Read the model definition and answer for the solid it produces. Units are mm, in the model's axes. Give positions to 0.01 mm unless a question says otherwise; leave off trailing zeros. Order: outer loops, then holes, each group sorted by start corner. A loop starts at its lowest first (then second) coordinate and runs counter-clockwise, first axis right, second up. Notation, with made-up numbers: M 41.25,10.5 L 93.25,10.5 A32 ccw 93.25,45.5 Z; hole C 23,79 d3. An arc over 180 degrees is marked long. Write item = value, one per line. Start each with the question number.
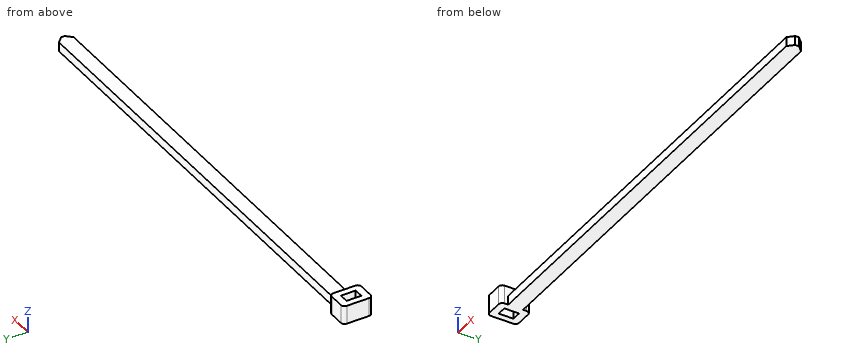
from build123d import *

# Parameters (mm, degrees)
F0_W     = 100
F0_H     = 3.2
F1_DEPTH = 2
F2_SIZE  = 1.2
F3_W     = 4.8
F3_H     = 6.4
F3_W_2   = 2
F3_H_2   = 3.2
F4_DEPTH = 4
F5_R     = 0.8


with BuildPart() as f1:
    # F0 (on Top) → F1 (new body)
    with BuildSketch(Plane.XY):
        Rectangle(F0_W, F0_H)
    extrude(amount=F1_DEPTH)

    # F2
    f2_edges = [f1.edges().sort_by_distance(p)[0] for p in [
        (50, 1.6, 1),
        (50, -1.6, 1),
    ]]
    chamfer(f2_edges, length=F2_SIZE)

    # F3 (on Top) → F4 (join)
    with BuildSketch(Plane.XY):
        with Locations((-52.4, 0)):
            Rectangle(F3_W, F3_H)
        with Locations((-52.4, 0)):
            Rectangle(F3_W_2, F3_H_2, mode=Mode.SUBTRACT)
    extrude(amount=F4_DEPTH)

    # F5
    f5_edges = [f1.edges().sort_by_distance(p)[0] for p in [
        (-54.8, 3.2, 2),
        (-50, 3.2, 2),
        (-50, -3.2, 2),
        (-54.8, -3.2, 2),
    ]]
    fillet(f5_edges, radius=F5_R)


solid = f1.part
1) Find section B-B on x = 23. Determine the outline of the cut face in (y, z), plus the area to 3 significant figures.
2) Find section A-A on z = 3.2. Determine the outline of the cut face in (x, y), plus the area to 3 significant figures.
3) Each of these flat-tipped pins is pushed along its axis until it touches: P1, Ø1, axis at x = 6, y = -0.5, coming from the +Z side; P2, Ø1, axis at x = 21, z = 0.5, coming from the -Y side; P3, Ø2, axis at x = -25, z = 1, coming from the +Y side. Where does it stop, or does it pass through?
4) Find the intervals of material crossed by probe 1 along X at (y, z) = (0.25, 1.2); probe 2 along X at (y, z) = (-0.5, 2.45); probe 3 along Y at (x, z) = (21.5, 1.15), in increasing order. Write a range as [from, to].
Numbers:
q1.outline = M -1.6,0 L 1.6,0 L 1.6,2 L -1.6,2 Z
q1.area = 6.40 mm2
q2.outline = M -54.8,-2.4 A0.8 ccw -54,-3.2 L -50.8,-3.2 A0.8 ccw -50,-2.4 L -50,2.4 A0.8 ccw -50.8,3.2 L -54,3.2 A0.8 ccw -54.8,2.4 Z; hole M -53.4,-1.6 L -51.4,-1.6 L -51.4,1.6 L -53.4,1.6 Z
q2.area = 23.8 mm2
q3.P1 = 2
q3.P2 = -1.6
q3.P3 = 1.6
q4.probe_1 = [-54.8, -53.4], [-51.4, 50]
q4.probe_2 = [-54.8, -53.4], [-51.4, -50]
q4.probe_3 = [-1.6, 1.6]
